Geometry check sheet. Reference: the model listing, model coordinates, mm. A direction names the side the tool comes from. Coordinates: 2 decimals unless noted, no trailing zeros. Write each loop counter-clockwise with the first axis right and the second up, starting at its lowest first coordinate (ties: lowest second). Pieces come first, ordered by that corner, then holes. Notation, with made-up numbers: (31, 25.5) -> (51, 25.5) arc R9 ccw to (51, 34.5) -> close; hole circle Ø4 at (38.5, -1). An arc over 180 degrees is marked (long way). One line per question, with ' | ' between items.
from build123d import *

# Parameters (mm, degrees)
BOSS_EXTRUDE1_DEPTH      = 10
BOSS_EXTRUDE1_DEPTH_BACK = 0.01
SKETCH3_W                = 38
SKETCH3_H                = 54
CUT_EXTRUDE1_DEPTH       = 3
SKETCH5_W                = 38
SKETCH5_H                = 54
CUT_EXTRUDE3_DEPTH       = 3
SKETCH7_W                = 54
SKETCH7_H                = 165
CUT_EXTRUDE4_DEPTH       = 6.5
SKETCH15_W               = 20
SKETCH15_H               = 50
BOSS_EXTRUDE3_DEPTH      = 20.3
SKETCH18_W               = 43.4
SKETCH18_H               = 43.4
CUT_EXTRUDE18_DEPTH      = 3
SKETCH21_R               = 9
CUT_EXTRUDE21_DEPTH      = 20
SKETCH22_R               = 1.55
CUT_EXTRUDE23_DEPTH      = 223.739666272
SKETCH25_W               = 59
SKETCH25_H               = 8.1
BOSS_EXTRUDE5_DEPTH      = 3.5
SKETCH28_W               = 4.75290021
SKETCH28_H               = 9.947843747
BOSS_EXTRUDE6_DEPTH      = 141.870057685
SKETCH36_W               = 38
SKETCH36_H               = 2
BOSS_EXTRUDE7_DEPTH      = 37
SKETCH39_R               = 6
SKETCH39_R_2             = 1.55
CUT_EXTRUDE28_DEPTH      = 2
SKETCH42_R               = 6
SKETCH42_R_2             = 1.55
CUT_EXTRUDE29_DEPTH      = 2
SKETCH44_W               = 2.25
SKETCH44_H               = 7.82
CUT_EXTRUDE30_DEPTH      = 59
BOSS_EXTRUDE8_REACH      = 227.847
SKETCH45_W               = 16.5
SKETCH45_H               = 32
SKETCH30_W               = 14.12
SKETCH30_H               = 25
CUT_EXTRUDE25_DEPTH      = 4.5
SKETCH33_R               = 1.55
CUT_EXTRUDE26_DEPTH      = 10.017641697
SKETCH46_R               = 5
CUT_EXTRUDE31_DEPTH      = 225.11173314
SKETCH47_W               = 6.139074003
SKETCH47_H               = 38.880802014
SKETCH47_W_2             = 4.706623401
SKETCH47_H_2             = 54.433122819
SKETCH47_W_3             = 4.092716002
SKETCH47_H_3             = 31.923184811
CUT_EXTRUDE32_DEPTH      = 225.11173314


with BuildPart() as part:
    # Sketch1 → Boss-Extrude1 (new, two sides: drawn at the far end of the back side and taken through both)
    with BuildSketch(Plane.XY.offset(-BOSS_EXTRUDE1_DEPTH_BACK)):
        with BuildLine():
            Line((0, 0), (0, -50))
            Line((0, -50), (60, -50))
            Line((60, -50), (60, -65))
            Line((60, -65), (33.129942315, -91.870057685))
            Line((33.129942315, -91.870057685), (-55.850057685, -91.870057685))
            ThreePointArc((-55.850057685, -91.870057685), (-147.4724214, -76.71648961), (-199.999956277, -0.132246858))
            ThreePointArc((-199.999956277, -0.132246858), (-147.567879237, 76.64550452), (-55.850057685, 91.870057685))
            Line((-55.850057685, 91.870057685), (33.129942315, 91.870057685))
            Line((33.129942315, 91.870057685), (60, 65))
            Line((60, 65), (60, 50))
            Line((60, 50), (0, 50))
            Line((0, 50), (0, 0))
        make_face()
    extrude(amount=BOSS_EXTRUDE1_DEPTH + BOSS_EXTRUDE1_DEPTH_BACK)

    # Sketch3 → Cut-Extrude1 (cut)
    with BuildSketch(Plane.XY.offset(10)):
        with Locations((-19, 64.870057685)):
            Rectangle(SKETCH3_W, SKETCH3_H)
    extrude(amount=-CUT_EXTRUDE1_DEPTH, mode=Mode.SUBTRACT)

    # Sketch5 → Cut-Extrude3 (cut)
    with BuildSketch(Plane.XY.offset(10)):
        with Locations((-19, -64.870057685)):
            Rectangle(SKETCH5_W, SKETCH5_H)
    extrude(amount=-CUT_EXTRUDE3_DEPTH, mode=Mode.SUBTRACT)

    # Sketch7 → Cut-Extrude4 (cut)
    with BuildSketch(Plane.XY.offset(10)):
        with Locations((-66.32515636, 0.28573122)):
            Rectangle(SKETCH7_W, SKETCH7_H)
    extrude(amount=-CUT_EXTRUDE4_DEPTH, mode=Mode.SUBTRACT)

    # Sketch15 → Boss-Extrude3 (add)
    with BuildSketch(Plane.XY.offset(10)):
        with Locations((-10, 0.20156489)):
            Rectangle(SKETCH15_W, SKETCH15_H)
    extrude(amount=BOSS_EXTRUDE3_DEPTH)

    # Sketch18 → Cut-Extrude18 (cut)
    with BuildSketch(Plane.XY.offset(10)):
        with Locations((-123.42454895, 39.3)):
            Rectangle(SKETCH18_W, SKETCH18_H)
    extrude(amount=-CUT_EXTRUDE18_DEPTH, mode=Mode.SUBTRACT)

    # Sketch21 → Cut-Extrude21 (cut)
    with BuildSketch(Plane(origin=(0, 0, 0), x_dir=(0, 0, -1), z_dir=(1, 0, 0))):
        with Locations((-19.36187505, 12.37175029)):
            Circle(SKETCH21_R)
        with Locations((-19.26539558, -14.62824971)):
            Circle(SKETCH21_R)
        with BuildLine():
            Line((-9.491579533, 2.276446619), (-9.557448357, -4.178698144))
            ThreePointArc((-9.557448357, -4.178698144), (-12.081396215, -6.651657156), (-14.554355227, -4.127709299))
            Line((-14.554355227, -4.127709299), (-14.488486403, 2.327435464))
            ThreePointArc((-14.488486403, 2.327435464), (-11.964538545, 4.800394476), (-9.491579533, 2.276446619))
        make_face()
    extrude(amount=-CUT_EXTRUDE21_DEPTH, mode=Mode.SUBTRACT)

    # Sketch22 → Cut-Extrude23 (cut, through all)
    with BuildSketch(Plane.XY.offset(7)):
        with Locations((-143.16862044, 58.97947337)):
            Circle(SKETCH22_R)
        with Locations((-103.76862044, 58.97947337)):
            Circle(SKETCH22_R)
        with Locations((-103.76862044, 19.57947337)):
            Circle(SKETCH22_R)
        with Locations((-143.16862044, 19.57947337)):
            Circle(SKETCH22_R)
    extrude(amount=-CUT_EXTRUDE23_DEPTH, mode=Mode.SUBTRACT)

    # Sketch25 → Boss-Extrude5 (add)
    with BuildSketch(Plane.XY.offset(10)):
        with Locations((-133.432578579, -2.134090808)):
            Rectangle(SKETCH25_W, SKETCH25_H)
    extrude(amount=BOSS_EXTRUDE5_DEPTH)

    # Sketch28 → Boss-Extrude6 (add)
    with BuildSketch(Plane.XZ.offset(91.870057685)):
        with Locations((16.603067585, 5.033719824)):
            Rectangle(SKETCH28_W, SKETCH28_H)
    extrude(amount=-BOSS_EXTRUDE6_DEPTH)

    # Sketch36 → Boss-Extrude7 (add)
    with BuildSketch(Plane.XY.offset(7)):
        Polygon((0.325623195, 91.814547745), (0.318530176, 89.814560323), (-37.681230846, 89.949327676), (-37.674137828, 91.949315098), align=None)
        with Locations((-19, -90.81512516)):
            Rectangle(SKETCH36_W, SKETCH36_H)
    extrude(amount=BOSS_EXTRUDE7_DEPTH)

    # Sketch39 → Cut-Extrude28 (cut)
    with BuildSketch(Plane.XZ.offset(91.81512516)):
        with Locations(Location((-19, 19, 0), (0, 0, 270))):
            Circle(SKETCH39_R)
        with Locations(Location((-34.499611559, 25.01055106, 0), (0, 0, 270))):
            Circle(SKETCH39_R_2)
        with Locations(Location((-3.563871147, 24.988758691, 0), (0, 0, 270))):
            Circle(SKETCH39_R_2)
        with Locations(Location((-28.819186805, 37.01055106, 0), (0, 0, 270))):
            Circle(SKETCH39_R_2)
        with Locations(Location((-9.177448314, 36.988758691, 0), (0, 0, 270))):
            Circle(SKETCH39_R_2)
        with Locations(Location((-28.819994175, 13.01055106, 0), (0, 0, 270))):
            Circle(SKETCH39_R_2)
        with Locations(Location((-9.230494356, 12.988758691, 0), (0, 0, 270))):
            Circle(SKETCH39_R_2)
    extrude(amount=-CUT_EXTRUDE28_DEPTH, mode=Mode.SUBTRACT)

    # Sketch42 → Cut-Extrude29 (cut)
    with BuildSketch(Plane(origin=(0.325623195, 91.814547745, 0), x_dir=(0.9999937111161443, -0.003546509292438372, 0), z_dir=(0.003546509292438372, 0.9999937111161443, 0))):
        with Locations(Location((-19.325818013, -19, 0), (0, 0, 180))):
            Circle(SKETCH42_R)
        with Locations(Location((-29.070149337, -13, 0), (0, 0, 180))):
            Circle(SKETCH42_R_2)
        with Locations(Location((-3.778432466, -25, 0), (0, 0, 180))):
            Circle(SKETCH42_R_2)
        with Locations(Location((-9.464104196, -13, 0), (0, 0, 180))):
            Circle(SKETCH42_R_2)
        with Locations(Location((-34.772326096, -25, 0), (0, 0, 180))):
            Circle(SKETCH42_R_2)
        with Locations(Location((-29.096493177, -37, 0), (0, 0, 180))):
            Circle(SKETCH42_R_2)
        with Locations(Location((-9.473371075, -37, 0), (0, 0, 180))):
            Circle(SKETCH42_R_2)
    extrude(amount=-CUT_EXTRUDE29_DEPTH, mode=Mode.SUBTRACT)

    # Sketch44 → Cut-Extrude30 (cut)
    with BuildSketch(Plane.ZY.offset(162.932578579)):
        with Locations((11.13716849, -2.28119145)):
            Rectangle(SKETCH44_W, SKETCH44_H)
    extrude(amount=-CUT_EXTRUDE30_DEPTH, mode=Mode.SUBTRACT)

    # Boss-Extrude8: up to this face of the body (flat: up to its plane)
    boss_extrude8_end = Plane(part.part.faces().sort_by_distance((16.603067585, -20.935028843, 10.007641697))[0])
    # Sketch45 → Boss-Extrude8 (add, up to the picked face)
    with BuildSketch(Plane(origin=(0, 0, -0.01), x_dir=(-1, 0, 0), z_dir=(0, 0, -1)), mode=Mode.PRIVATE) as boss_extrude8_sk1:
        Polygon((-0.170650113, 17.999191052), (-0.474028092, 49.997752923), (-16.973286556, 49.841323653), (-16.669908578, 17.842761782), align=None)
    boss_extrude8_tool1 = split(extrude(boss_extrude8_sk1.sketch, amount=-BOSS_EXTRUDE8_REACH, mode=Mode.PRIVATE), bisect_by=boss_extrude8_end, keep=Keep.BOTH, mode=Mode.PRIVATE)
    # Sketch45 → Boss-Extrude8 (add, up to the picked face)
    with BuildSketch(Plane(origin=(0, 0, -0.01), x_dir=(-1, 0, 0), z_dir=(0, 0, -1)), mode=Mode.PRIVATE) as boss_extrude8_sk2:
        with Locations((-8.25, -34)):
            Rectangle(SKETCH45_W, SKETCH45_H)
    boss_extrude8_tool2 = split(extrude(boss_extrude8_sk2.sketch, amount=-BOSS_EXTRUDE8_REACH, mode=Mode.PRIVATE), bisect_by=boss_extrude8_end, keep=Keep.BOTH, mode=Mode.PRIVATE)
    add(boss_extrude8_tool1.solids().sort_by(Axis((8.571968, 33.920257, -0.01), (0, 0, 1)))[0])
    add(boss_extrude8_tool2.solids().sort_by(Axis((8.25, -34, -0.01), (0, 0, 1)))[0])

    # Sketch30 → Cut-Extrude25 (cut)
    with BuildSketch(Plane(origin=(0, 0, -0.01), x_dir=(-1, 0, 0), z_dir=(0, 0, -1))):
        with Locations((-7.06, -28.51)):
            Rectangle(SKETCH30_W, SKETCH30_H)
        Polygon((-14.292411252, 40.945582253), (-14.187225928, 15.945803533), (-0.067350907, 16.005212204), (-0.172536231, 41.004990924), align=None)
    extrude(amount=-CUT_EXTRUDE25_DEPTH, mode=Mode.SUBTRACT)

    # Sketch33 → Cut-Extrude26 (cut)
    with BuildSketch(Plane(origin=(0, 0, -0.01), x_dir=(-1, 0, 0), z_dir=(0, 0, -1))):
        with Locations((-7.06, -33)):
            Circle(SKETCH33_R)
        with Locations((-7.06, -29)):
            Circle(SKETCH33_R)
        with Locations((-7.06, -25)):
            Circle(SKETCH33_R)
        with Locations((-7.06, -21)):
            Circle(SKETCH33_R)
        with Locations((-7.145509491, 20.971058488)):
            Circle(SKETCH33_R)
        with Locations((-7.161808177, 24.971025282)):
            Circle(SKETCH33_R)
        with Locations((-7.178106862, 28.970992076)):
            Circle(SKETCH33_R)
        with Locations((-7.194405548, 32.97095887)):
            Circle(SKETCH33_R)
    extrude(amount=-CUT_EXTRUDE26_DEPTH, mode=Mode.SUBTRACT)

    # Sketch46 → Cut-Extrude31 (cut, through all)
    with BuildSketch(Plane.XY.offset(10)):
        with Locations((-32, 28)):
            Circle(SKETCH46_R)
        with Locations((-32, 14)):
            Circle(SKETCH46_R)
        with Locations((-32, 0)):
            Circle(SKETCH46_R)
        with Locations((-32, -14)):
            Circle(SKETCH46_R)
        with Locations((-32, -28)):
            Circle(SKETCH46_R)
    extrude(amount=-CUT_EXTRUDE31_DEPTH, mode=Mode.SUBTRACT)

    # Sketch47 → Cut-Extrude32 (cut, through all)
    with BuildSketch(Plane.XY.offset(10)):
        with Locations((-164.132446172, 28.036052806)):
            Rectangle(SKETCH47_W, SKETCH47_H)
        with Locations((-98.546672249, -38.879853818)):
            Rectangle(SKETCH47_W_2, SKETCH47_H_2)
        with Locations((-169.043705373, -29.057335414)):
            Rectangle(SKETCH47_W_3, SKETCH47_H_3)
    extrude(amount=-CUT_EXTRUDE32_DEPTH, mode=Mode.SUBTRACT)


solid = part.part
1. Tool access check on faces 1 (the face through (-19, -63, 7)), 2 (the face through (-36, 25, 5)). Record the directions out of +Z, -Z, +X, -X, +Y, -Y that give a thin tool (end or side, any length) a straight path to the whole face; none if there is none.
Worked answers:
face 1: +Z | face 2: +Z, -Z
2. Cross-section at A-A on x = -64.5. Record the boundary of the cut face in (y, z), and give its area (3 significant figures).
Worked answers:
outline: (-93.64, -0.01) -> (93.64, -0.01) -> (93.64, 10) -> (82.79, 10) -> (82.79, 3.5) -> (-82.21, 3.5) -> (-82.21, 10) -> (-93.64, 10) -> close | area: 802 mm²
3. Material ranges on line 1 (Y direction, x = -32, z = 2.75); line 2 (X direction, y = -40.5, z = 8.5); line 3 (Y direction, x = -26, z = 25), recorded low to high. Write a range as from..to.
Worked answers:
line 1: -91.87..-33, -23..-19, -9..-5, 5..9, 19..23, 33..91.87 | line 2: -183.73..-171.09, -167..-100.9, -96.19..-93.33, -39.33..-38, 0..18.98 | line 3: -91.82..-89.82, 89.91..91.91
4. Cross-section at B-B on y = 73. Record the boundary of the cut face in (x, z), and give its area (3 significant figures).
Worked answers:
outline: (-152.95, -0.01) -> (52, -0.01) -> (52, 10) -> (0, 10) -> (0, 7) -> (-38, 7) -> (-38, 10) -> (-39.33, 10) -> (-39.33, 3.5) -> (-93.33, 3.5) -> (-93.33, 10) -> (-152.95, 10) -> close | area: 1,590 mm²
5. Mould release check, pull along X, two halves, no side actions. Record for faces 3 (the face through (9, 30, 4.49)), 4 (the face through (-134, -2, 13.5)): released by +X, released by -X, zero draft, split by the parting line, or undercut.
Worked answers:
face 3: undercut | face 4: zero draft
6. Go/stop test with flat-tipped pins: P1, Ø2, axis at y = -30.5, z = 6, coming from the +X side; P2, Ø2.5, axis at x = -98, z = 4.5, coming from the -Y side; P3, Ø19, axis at x = -14, y = -68, coming from the +Z side. Record where each tip stops, or that it passes through.
Worked answers:
P1: x = 18.98 | P2: y = -94.53 | P3: z = 7
